from build123d import *

# Parameters (mm, degrees)
F0_R     = 10
F1_DEPTH = 4
F2_D     = 5


# Not quite as in the source:
# - a feature names something its author has since deleted; it is built from what else it names
# - the program builds the solid bodies; features that only make, move or delete a surface that nothing else refers to are left out


with BuildPart() as f1:
    # F0 (on Top) → F1 (new body)
    with BuildSketch(Plane.XY):
        Polygon((1.9552472353, 143.8201326668), (-96.4947527647, 143.8201326668), (-96.4947527647, -33.5798673332), (1.9552472353, -33.5798673332), (1.9552472353, -26.5798673332), (12.4552472353, -26.5798673332), (12.4552472353, -33.5798673332), (110.9052472353, -33.5798673332), (110.9052472353, 143.8201326668), (12.4552472353, 143.8201326668), (12.4552472353, 136.8201326668), (1.9552472353, 136.8201326668), align=None)
        with Locations((-66.4946527647, -3.5798663332)):
            Circle(F0_R, mode=Mode.SUBTRACT)
        with Locations((-17.3613527647, -3.5798663332)):
            Circle(F0_R, mode=Mode.SUBTRACT)
        with Locations((-66.4946527647, 35.5534666668)):
            Circle(F0_R, mode=Mode.SUBTRACT)
        with Locations((-17.3613527647, 35.5534666668)):
            Circle(F0_R, mode=Mode.SUBTRACT)
        with Locations((31.7719472353, -3.5798663332)):
            Circle(F0_R, mode=Mode.SUBTRACT)
        with Locations((80.9052472353, -3.5798663332)):
            Circle(F0_R, mode=Mode.SUBTRACT)
        with Locations((31.7719472353, 35.5534666668)):
            Circle(F0_R, mode=Mode.SUBTRACT)
        with Locations((80.9052472353, 35.5534666668)):
            Circle(F0_R, mode=Mode.SUBTRACT)
        with Locations((-66.4946527647, 74.6867996668)):
            Circle(F0_R, mode=Mode.SUBTRACT)
        with Locations((-17.3613527647, 74.6867996668)):
            Circle(F0_R, mode=Mode.SUBTRACT)
        with Locations((-66.4946527647, 113.8201326668)):
            Circle(F0_R, mode=Mode.SUBTRACT)
        with Locations((-17.3613527647, 113.8201326668)):
            Circle(F0_R, mode=Mode.SUBTRACT)
        with Locations((31.7719472353, 74.6867996668)):
            Circle(F0_R, mode=Mode.SUBTRACT)
        with Locations((80.9052472353, 74.6867996668)):
            Circle(F0_R, mode=Mode.SUBTRACT)
        with Locations((31.7719472353, 113.8201326668)):
            Circle(F0_R, mode=Mode.SUBTRACT)
        with Locations((80.9052472353, 113.8201326668)):
            Circle(F0_R, mode=Mode.SUBTRACT)
    extrude(amount=F1_DEPTH)

    # F2 (through all)
    with Locations(Plane(origin=(0, 0, 0), x_dir=(1, 0, 0), z_dir=(0, 0, -1))):
        with Locations((18.5052472353, -55.1201326668), (-11.4947527647, -55.1201326668), (-56.4947527647, -55.1201326668), (93.5052472353, -55.1201326668), (-26.4947527647, -55.1201326668), (78.5052472353, -55.1201326668), (63.5052472353, -55.1201326668), (-71.4947527647, -55.1201326668), (33.5052472353, -55.1201326668), (-41.4947527647, -55.1201326668), (3.5052472353, -55.1201326668), (48.5052472353, -55.1201326668), (-86.4947527647, -55.1201326668)):
            Hole(F2_D / 2)


solid = f1.part
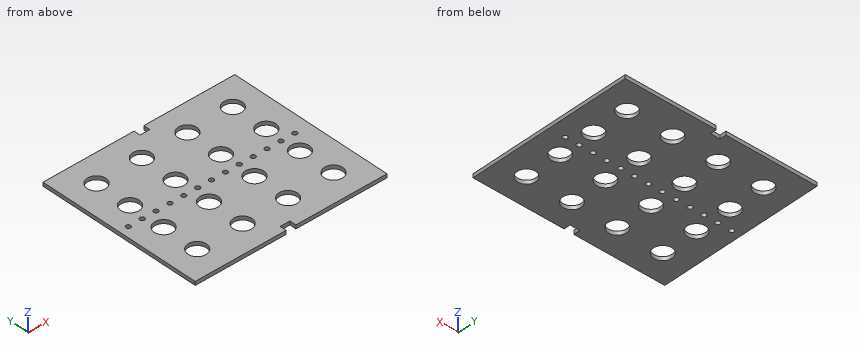
CAD build for the part. Positions are in the model's coordinates, mm. Round coordinates to 2 decimals unless told otherwise and drop trailing zeros. Order: outer loops, then holes, each group sorted by start corner. A loop starts at its lowest first (then second) coordinate and runs counter-clockwise, first axis right, second up. Notation, with made-up numbers: (-8, 21) - (0, 21) arc R11 ccw to (0, 40) - close; hole circle Ø1 at (57.25, 47.25). An arc over 180 degrees is marked (long way). Return JSON: item names as keys, results as strings.
(1) Wall check: probe 1 along Y at (x, z) = (76.5, 0.5); probe 2 along Y at (x, z) = (3, 1.4); probe 3 along X at (y, z) = (-12.5, 2.2). Give the ranges that are in metal, low to high. Write a range as from..to.
Answer key:
{"probe 1": "y = -33.58..-12.56, 5.4..26.58, 44.53..53.63, 56.61..65.71, 83.66..104.84, 122.8..143.82", "probe 2": "y = -26.58..52.67, 57.57..136.82", "probe 3": "x = -96.49..-71.01, -61.97..-21.88, -12.84..27.25, 36.29..76.39, 85.43..110.91"}
(2) Cut at D-D (z = 1.45). State how many separate pieces and enclosed holes the cut face has, then the cut area to 3 significant figures.
Answer key:
{"separate pieces": "1", "enclosed holes": "29", "area": "31,400 mm^2"}
(3) Pin check, flat tips, straight feed: pin 1 Ø18 at (x, y) = (-17.36, -3.58) entering from -Z; pin 2 Ø1 at (x, y) = (65.5, 103) entering from -Z; pin 3 Ø1.2 at (x, z) = (10, 3) entering from +Y. Stop position of each tip, or through.
Answer key:
{"pin 1": "passes through", "pin 2": "stops at z = 0", "pin 3": "stops at y = 136.82"}
(4) Cut at C-C (y = 78). Give the cut face in (x, z), then the cut area to 3 significant figures.
Answer key:
{"outline": "(-96.49, 0) - (-75.93, 0) - (-75.93, 4) - (-96.49, 4) - close; (-57.06, 0) - (-26.8, 0) - (-26.8, 4) - (-57.06, 4) - close; (-7.93, 0) - (22.34, 0) - (22.34, 4) - (-7.93, 4) - close; (41.21, 0) - (71.47, 0) - (71.47, 4) - (41.21, 4) - close; (90.34, 0) - (110.91, 0) - (110.91, 4) - (90.34, 4) - close", "area": "528 mm^2"}
(5) Cut at B-B (x = 78.5). Give the cut face in (y, z), then the cut area to 3 significant figures.
Answer key:
{"outline": "(-33.58, 0) - (-13.29, 0) - (-13.29, 4) - (-33.58, 4) - close; (6.13, 0) - (25.85, 0) - (25.85, 4) - (6.13, 4) - close; (45.26, 0) - (52.62, 0) - (52.62, 4) - (45.26, 4) - close; (57.62, 0) - (64.98, 0) - (64.98, 4) - (57.62, 4) - close; (84.39, 0) - (104.11, 0) - (104.11, 4) - (84.39, 4) - close; (123.53, 0) - (143.82, 0) - (143.82, 4) - (123.53, 4) - close", "area": "379 mm^2"}
(6) Cut at A-A (y = 28). Give the cut face in (x, z), then the cut area to 3 significant figures.
Answer key:
{"outline": "(-96.49, 0) - (-73.05, 0) - (-73.05, 4) - (-96.49, 4) - close; (-59.94, 0) - (-23.91, 0) - (-23.91, 4) - (-59.94, 4) - close; (-10.81, 0) - (25.22, 0) - (25.22, 4) - (-10.81, 4) - close; (38.33, 0) - (74.35, 0) - (74.35, 4) - (38.33, 4) - close; (87.46, 0) - (110.91, 0) - (110.91, 4) - (87.46, 4) - close", "area": "620 mm^2"}
